Check sheet for the drawn part. Datum: minimum x, y, z corner. Units: mm. A direction names the side the tool comes from. Give positions to 0.01 mm unless a question says otherwise; leave off trailing zeros. Write each loop counter-clockwise with the first axis right and the second up, starting at its lowest first coordinate (ties: lowest second). Pieces come first, ordered by that corner, then holes. Notation, with made-up numbers: M 24.25,21 L 60.25,21 A18 ccw 60.25,51 Z; hole C 30,-20.75 d3. An arc over 180 degrees is marked long. Use CSV: the item, a comma, the result in double quotes. Start each with the question number.
1. Cross-section at B-B, the plane x = 29. Enter the section's corners in (y, z).
2. Cross-section at C-C, the plane z = 35. Enter the section's corners in (x, y).
3. Mould release check, pull along Z, two halves, no side actions. Record for the marked faces 5, 6 and 7: +Z half, -Z half, draft (parallel to the pull), parting line (faces both ways), or undercut.
4. Access from +Z, -Z, +X, -X, +Y, -Y to the whole of each face (thin tool, end or side, straight path). Record for the marked faces 1, 2, 3 and 4.
5. Depth check by flat-ended pin: P1, Ø2, axis at x = 50, z = 63, coming from the +Y side; P2, Ø2, axis at x = 72.5, z = 65.5, coming from the +Y side; P3, Ø7, axis at y = 2.5, z = 36, coming from the +X side; P4, Ø0.9, axis at x = 54, y = 10.5, coming from the +Z side. Enter the tip coordinate at first touch or a pass-through.
6. Cross-section at A-A, the plane y = 4. Enter the section's corners in (x, z).
7. Scan lines: line 1 (X direction, y = 7.5, z = 4.5); line 2 (X direction, y = 7, z = 29); line 3 (X direction, y = 3, z = 28). Record each from-to range of solid material in increasing order.
8. Cross-section at D-D, the plane y = 10.25. Enter the section's corners in (x, z), and give its area (3 significant figures).
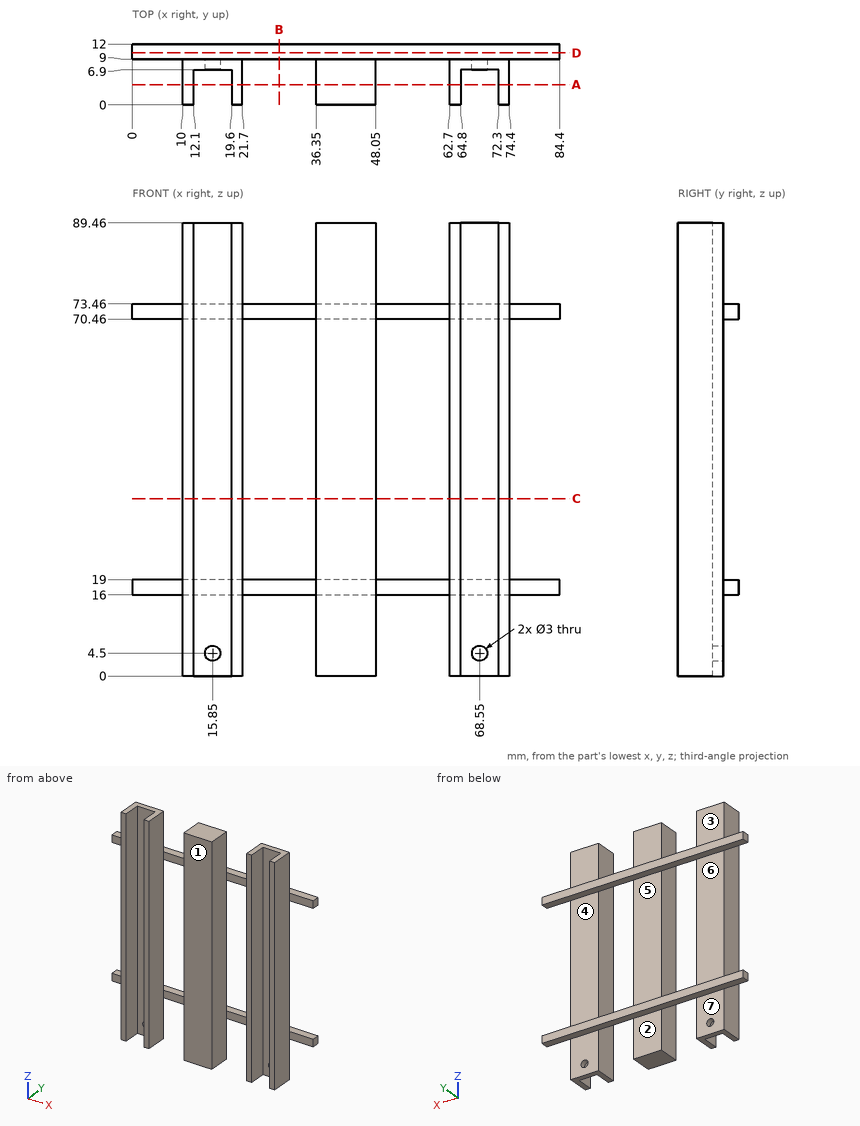
Worked answers:
1,outline,"M 9,16 L 12,16 L 12,19 L 9,19 Z; M 9,70.46 L 12,70.46 L 12,73.46 L 9,73.46 Z"
2,outline,"M 10,0 L 12.1,0 L 12.1,6.9 L 19.6,6.9 L 19.6,0 L 21.7,0 L 21.7,9 L 10,9 Z; M 36.35,0 L 48.05,0 L 48.05,9 L 36.35,9 Z; M 62.7,0 L 64.8,0 L 64.8,6.9 L 72.3,6.9 L 72.3,0 L 74.4,0 L 74.4,9 L 62.7,9 Z"
3,face 5,"undercut"
3,face 6,"undercut"
3,face 7,"draft"
4,face 1,"+Z, -Z, +X, -X, -Y"
4,face 2,"-Z, +X, -X, +Y"
4,face 3,"+Z, +X, -X, +Y"
4,face 4,"+X, -X, +Y"
5,P1,"passes through"
5,P2,"stops at y = 9"
5,P3,"stops at x = 74.4"
5,P4,"stops at z = 73.46"
6,outline,"M 10,0 L 12.1,0 L 12.1,89.46 L 10,89.46 Z; M 19.6,0 L 21.7,0 L 21.7,89.46 L 19.6,89.46 Z; M 36.35,0 L 48.05,0 L 48.05,89.46 L 36.35,89.46 Z; M 62.7,0 L 64.8,0 L 64.8,89.46 L 62.7,89.46 Z; M 72.3,0 L 74.4,0 L 74.4,89.46 L 72.3,89.46 Z"
7,line 1,"x = 10 to 14.35, 17.35 to 21.7, 36.35 to 48.05, 62.7 to 67.05, 70.05 to 74.4"
7,line 2,"x = 10 to 21.7, 36.35 to 48.05, 62.7 to 74.4"
7,line 3,"x = 10 to 12.1, 19.6 to 21.7, 36.35 to 48.05, 62.7 to 64.8, 72.3 to 74.4"
8,outline,"M 0,16 L 84.4,16 L 84.4,19 L 0,19 Z; M 0,70.46 L 84.4,70.46 L 84.4,73.46 L 0,73.46 Z"
8,area,"506 mm^2"
